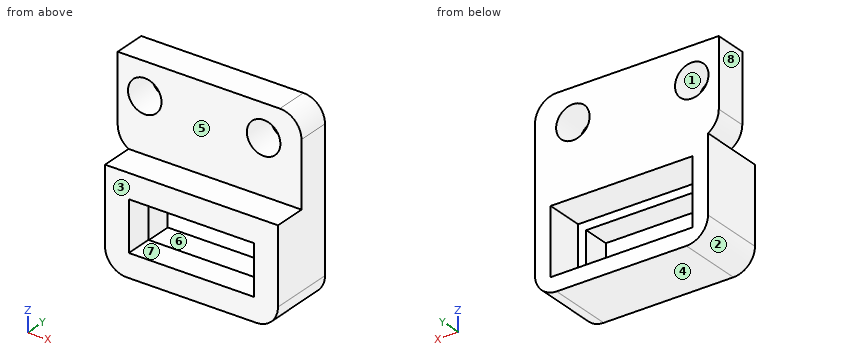
```python
from build123d import *

# Parameters (mm, degrees)
CROQUIS1_W              = 18
CROQUIS1_H              = 18
CROQUIS1_R              = 1.55
SALIENTE_EXTRUIR1_DEPTH = 3
CROQUIS3_W              = 18
CROQUIS3_H              = 10
SALIENTE_EXTRUIR3_DEPTH = 3
CORTAR_EXTRUIR1_REACH   = 28.153
CROQUIS4_W              = 2
CROQUIS4_H              = 10
CROQUIS7_W              = 13.1
CROQUIS7_H              = 6.1
CORTAR_EXTRUIR2_DEPTH   = 6
CROQUIS9_W              = 16
CROQUIS9_H              = 10
CROQUIS9_W_2            = 13.1
CROQUIS9_H_2            = 6.1
SALIENTE_EXTRUIR4_DEPTH = 3
CROQUIS10_W             = 13.1
CROQUIS10_H             = 6.1
CROQUIS10_W_2           = 11.6
CROQUIS10_H_2           = 4.6
SALIENTE_EXTRUIR6_DEPTH = 2.5
CROQUIS11_W             = 16
CROQUIS11_H             = 1
CORTAR_EXTRUIR4_DEPTH   = 9
REDONDEO1_R             = 2
CROQUIS12_W             = 8
CROQUIS12_H             = 3
CORTAR_EXTRUIR5_DEPTH   = 1
CROQUIS14_W             = 16
CROQUIS14_H             = 3
CORTAR_EXTRUIR6_DEPTH   = 9
REDONDEO2_R             = 2


with BuildPart() as part:
    # Croquis1 → Saliente-Extruir1 (new body)
    with BuildSketch(Plane(origin=(0, 0, 0), x_dir=(1, 0, 0), z_dir=(0, 1, 0))):
        with Locations((9, 9)):
            Rectangle(CROQUIS1_W, CROQUIS1_H)
        with Locations(Location((3.5, 3, 0), (0, 0, 270))):
            Circle(CROQUIS1_R, mode=Mode.SUBTRACT)
        with Locations(Location((14.5, 3, 0), (0, 0, 270))):
            Circle(CROQUIS1_R, mode=Mode.SUBTRACT)
    extrude(amount=SALIENTE_EXTRUIR1_DEPTH)

    # Croquis3 → Saliente-Extruir3 (add)
    with BuildSketch(Plane(origin=(0, 3, 0), x_dir=(1, 0, 0), z_dir=(0, 1, 0))):
        with Locations((9, 13)):
            Rectangle(CROQUIS3_W, CROQUIS3_H)
    extrude(amount=SALIENTE_EXTRUIR3_DEPTH)

    # Cortar-Extruir1: up to this face of the body (flat: up to its plane)
    cortar_extruir1_end = Plane(part.part.faces().sort_by_distance((9, 6, -13))[0])
    # Croquis4 → Cortar-Extruir1 (cut, up to the picked face)
    with BuildSketch(Plane.XZ, mode=Mode.PRIVATE) as cortar_extruir1_sk1:
        with Locations((1, -13)):
            Rectangle(CROQUIS4_W, CROQUIS4_H)
    cortar_extruir1_tool1 = split(extrude(cortar_extruir1_sk1.sketch, amount=-CORTAR_EXTRUIR1_REACH, mode=Mode.PRIVATE), bisect_by=cortar_extruir1_end, keep=Keep.BOTH, mode=Mode.PRIVATE)
    add(cortar_extruir1_tool1.solids().sort_by(Axis((1, 0, -13), (0, 1, 0)))[0], mode=Mode.SUBTRACT)

    # Croquis7 → Cortar-Extruir2 (cut)
    with BuildSketch(Plane(origin=(0, 6, 0), x_dir=(1, 0, 0), z_dir=(0, 1, 0))):
        with Locations((10, 12.55)):
            Rectangle(CROQUIS7_W, CROQUIS7_H)
    extrude(amount=-CORTAR_EXTRUIR2_DEPTH, mode=Mode.SUBTRACT)

    # Croquis9 → Saliente-Extruir4 (add)
    with BuildSketch(Plane.XZ):
        with Locations((10, -13)):
            Rectangle(CROQUIS9_W, CROQUIS9_H)
        with Locations((10, -12.55)):
            Rectangle(CROQUIS9_W_2, CROQUIS9_H_2, mode=Mode.SUBTRACT)
    extrude(amount=SALIENTE_EXTRUIR4_DEPTH)

    # Croquis10 → Saliente-Extruir6 (add)
    with BuildSketch(Plane.XZ.offset(3)):
        with Locations((10, -12.55)):
            Rectangle(CROQUIS10_W, CROQUIS10_H)
        with Locations((10, -12.55)):
            Rectangle(CROQUIS10_W_2, CROQUIS10_H_2, mode=Mode.SUBTRACT)
    extrude(amount=-SALIENTE_EXTRUIR6_DEPTH)

    # Croquis11 → Cortar-Extruir4 (cut)
    with BuildSketch(Plane(origin=(0, 6, 0), x_dir=(1, 0, 0), z_dir=(0, 1, 0))):
        with Locations((10, 17.5)):
            Rectangle(CROQUIS11_W, CROQUIS11_H)
    extrude(amount=-CORTAR_EXTRUIR4_DEPTH, mode=Mode.SUBTRACT)

    # Redondeo1
    redondeo1_edges = [part.edges().sort_by_distance(p)[0] for p in [
        (18, 1.5, -17),
        (2, 1.5, -17),
        (18, 1.5, 0),
    ]]
    fillet(redondeo1_edges, radius=REDONDEO1_R)

    # Croquis12 → Cortar-Extruir5 (cut)
    with BuildSketch(Plane.ZY):
        with Locations((-4, 1.5)):
            Rectangle(CROQUIS12_W, CROQUIS12_H)
    extrude(amount=-CORTAR_EXTRUIR5_DEPTH, mode=Mode.SUBTRACT)

    # Croquis14 → Cortar-Extruir6 (cut)
    with BuildSketch(Plane.XY.offset(-8)):
        with Locations((10, 4.5)):
            Rectangle(CROQUIS14_W, CROQUIS14_H)
    extrude(amount=-CORTAR_EXTRUIR6_DEPTH, mode=Mode.SUBTRACT)

    # Redondeo2
    # the kernel refuses this fillet: 2 mm, written as the material it takes off along each edge
    with BuildSketch(Plane(origin=(1, 7.330127019, -8), x_dir=(0, 0, 1), z_dir=(0, -1, 0))) as redondeo2_piece_1:
        with BuildLine():
            CenterArc((1.732050808, -2), REDONDEO2_R, 90, 60)
            Line((0, -1), (-0.034641016, -0.98))
            ThreePointArc((-0.034641016, -0.98), (-0.04, -0.5), (-0.04, 0))
            Line((-0.04, 0), (0, 0.04))
            Line((0, 0.04), (1.732050808, 0.04))
            Line((1.732050808, 0.04), (1.732050808, 0))
        make_face()
    extrude(amount=11.660254038, mode=Mode.SUBTRACT)


solid = part.part
```
The model under review builds one solid part; all positions refer to its coordinate system, in mm. Face numbers are marked on the shaded views. A direction names the side the tool comes from. Give positions to 0.01 mm unless a question says otherwise; leave off trailing zeros. Loops run counter-clockwise (first coordinate to the right, second up) from the corner with the lowest first, then second, coordinate; pieces in that order, holes last. Notation, with made-up numbers: (-23.75, 60.5) - (23.25, 60.5) arc R32 ccw to (23.25, 91.5) - close; hole circle Ø5 at (44, 0). An arc over 180 degrees is marked (long way). Answer as a JSON object with one key per item and string values.
Q1. Add section C-C on x = 11.5. State the section outline as (y, z) points.
Worked out:
{"outline": "(-3, -17) - (3, -17) - (3, -15.6) - (-0.5, -15.6) - (-0.5, -14.85) - (-3, -14.85) - close; (-3, -10.25) - (-0.5, -10.25) - (-0.5, -9.5) - (3, -9.5) - (3, 0) - (0, 0) - (0, -8) - (-3, -8) - close"}
Q2. Add section D-D on y = 1.05. State the section outline as (x, z) points, plus the area to 3 significant figures.
Worked out:
{"outline": "(1, -6.27) arc R2 ccw to (2, -8) - (2, -15) arc R2 ccw to (4, -17) - (16, -17) arc R2 ccw to (18, -15) - (18, -2) arc R2 ccw to (16, 0) - (1, 0) - close; hole circle Ø3.1 at (3.5, -3); hole (3.45, -15.6) - (16.55, -15.6) - (16.55, -9.5) - (3.45, -9.5) - close; hole circle Ø3.1 at (14.5, -3)", "area": "182 mm^2"}
Q3. Add section A-A on z = -3. State the section outline as (x, y) points.
Worked out:
{"outline": "(1, 0) - (1.95, 0) - (1.95, 3) - (1, 3) - close; (5.05, 0) - (12.95, 0) - (12.95, 3) - (5.05, 3) - close; (16.05, 0) - (18, 0) - (18, 3) - (16.05, 3) - close"}
Q4. To check wall thickness, follow line 1 along X through (y, z) = (1.05, -3); line 2 along X through (y, z) = (-1.5, -12.25); line 3 along Z through (x, y) = (11, 1.5). State the ranges of each line that lie inside material, in increasing order.
Worked out:
{"line 1": "x = 1 to 1.95, 5.05 to 12.95, 16.05 to 18", "line 2": "x = 2 to 4.2, 15.8 to 18", "line 3": "z = -17 to -15.6, -9.5 to 0"}
Q5. Insertion check: pin 1 (0.8 mm diameter, centred on y = -1.5, z = -12.5, fed in from -X); pin 2 (9 mm diameter, centred on x = 11.5, z = -3, fed in from -Y); pin 3 (1.9 mm diameter, centred on x = 3.5, z = -3, fed in from +Y) (3 decimals); pin 4 (2.5 mm diameter, centred on x = 13, y = -1.5, fed in from +Z). Each pin has a flat end and moves straight along its axis. Give the tip position at first contact, or say it passes through.
Worked out:
{"pin 1": "stops at x = 2", "pin 2": "stops at y = 0", "pin 3": "passes through", "pin 4": "stops at z = -8"}
Q6. For the marked faces 4, 5, 6, 7 and 8, list the 3-axis set-ups (+Z, -Z, +X, -X, +Y, -Y) from which the entire face can be reached by the end or side of a thin tool; tool diameter is ignored.
Worked out:
{"face 4": "-Z, +X, -X, +Y, -Y", "face 5": "+Z, +X, -X, -Y", "face 6": "+Y", "face 7": "+Y, -Y", "face 8": "+Z, -Z, -X, +Y, -Y"}
Q7. Mouldability with a two-part tool opening along X and no side actions: class the marked faces 1, 2 and 3 as +X half, -X half, draft (parallel to the pull), parting line (faces both ways), or undercut.
Worked out:
{"face 1": "undercut", "face 2": "-X half", "face 3": "draft"}
Q8. Add section B-B on x = 14.5. State the section outline as (y, z) points.
Worked out:
{"outline": "(-3, -17) - (3, -17) - (3, -15.6) - (-0.5, -15.6) - (-0.5, -14.85) - (-3, -14.85) - close; (-3, -10.25) - (-0.5, -10.25) - (-0.5, -9.5) - (3, -9.5) - (3, -4.55) - (0, -4.55) - (0, -8) - (-3, -8) - close; (0, -1.45) - (3, -1.45) - (3, 0) - (0, 0) - close"}
